```python
from build123d import *

# Parameters (mm, degrees)
F1_DEPTH = 50


with BuildPart() as f1:
    # F0 (on Front) → F1 (new body, symmetric)
    with BuildSketch(Plane.XZ):
        with BuildLine():
            ThreePointArc((34.65832, 938.949756), (117.683363, 991.882101), (150, 1084.890842))
            ThreePointArc((150, 1084.890842), (-93.008741, 1202.574206), (-34.65832, 938.949756))
            ThreePointArc((-34.65832, 938.949756), (0, 934.890842), (34.65832, 938.949756))
        make_face()
        with BuildLine():
            ThreePointArc((34.65832, 938.949756), (0, 934.890842), (-34.65832, 938.949756))
            Line((-34.65832, 938.949756), (-34.65832, 414.451611))
            Line((-34.65832, 414.451611), (-496.485632, 782.202331))
            Line((-496.485632, 782.202331), (-577.730775, 697.129786))
            Line((-577.730775, 697.129786), (-34.65832, 364.602458))
            Line((-34.65832, 364.602458), (-34.65832, -64.047714))
            Line((-34.65832, -64.047714), (-456.351271, -622.056438))
            Line((-456.351271, -622.056438), (-399.381399, -665.109158))
            Line((-399.381399, -665.109158), (-34.65832, -182.486293))
            Line((-34.65832, -182.486293), (0, -136.624381))
            Line((0, -136.624381), (34.65832, -182.486293))
            Line((34.65832, -182.486293), (399.381399, -665.109158))
            Line((399.381399, -665.109158), (456.351271, -622.056438))
            Line((456.351271, -622.056438), (34.65832, -64.047714))
            Line((34.65832, -64.047714), (34.65832, 364.602458))
            Line((34.65832, 364.602458), (577.730775, 697.129786))
            Line((577.730775, 697.129786), (496.485632, 782.202331))
            Line((496.485632, 782.202331), (34.65832, 414.451611))
            Line((34.65832, 414.451611), (34.65832, 938.949756))
        make_face()
    extrude(amount=F1_DEPTH, both=True)


solid = f1.part
```
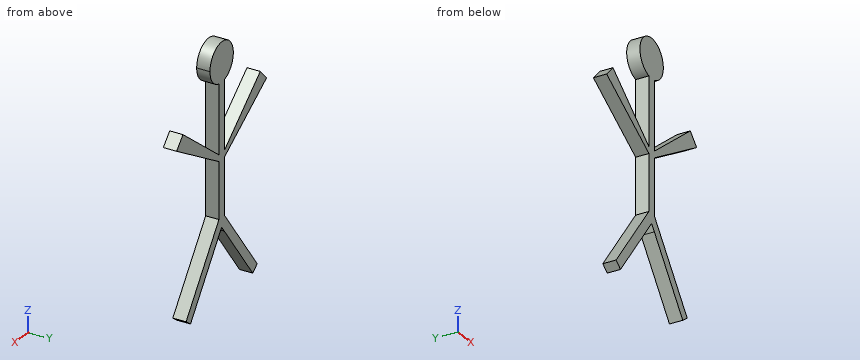
Geometry: final body of the model. Coordinates: model frame, mm. Round coordinates to 2 decimals unless told otherwise and drop trailing zeros. Order: outer loops, then holes, each group sorted by start corner. A loop starts at its lowest first (then second) coordinate and runs counter-clockwise, first axis right, second up. Notation, with made-up numbers: (32, 29.5) -> (37, 29.5) arc R28 cw to (37, 56.5) -> close; hole circle Ø3 at (-36.5, 19.5). An arc over 180 degrees is marked (long way). Write each question's results on one line, items separated by ' | '.
Q1. Ray query, line 1 along Z through (x, y) = (128, 3); line 2 along X through (y, z) = (10.5, 630); line 3 along Z through (x, y) = (-101.5, 37). Return the intervals inside material, ascending.
Response values:
line 1: -306 to -187.56, 421.76 to 488.78, 1006.69 to 1163.1 | line 2: -468.1 to -305.35, -34.66 to 34.66, 305.35 to 468.1 | line 3: -270.94 to -152.5, 405.53 to 467.68, 974.45 to 1195.33
Q2. Section query B-B (x = -420.5). Output: boundary loops of the cut face in (y, z).
Response values:
outline: (-50, -649.15) -> (50, -649.15) -> (50, -574.62) -> (-50, -574.62) -> close; (-50, 600.86) -> (50, 600.86) -> (50, 721.7) -> (-50, 721.7) -> close
Q3. Section query C-C (z = 457). Output: boundary loops of the cut face in (x, y), and give its area (3 significant figures).
Response values:
outline: (-185.56, -50) -> (-88.09, -50) -> (-88.09, 50) -> (-185.56, 50) -> close; (-34.66, -50) -> (34.66, -50) -> (34.66, 50) -> (-34.66, 50) -> close; (88.09, -50) -> (185.56, -50) -> (185.56, 50) -> (88.09, 50) -> close | area: 26,400 mm²
Q4. Section query D-D (y = 27.5). Output: boundary loops of the cut face in (x, z), and give its area (3 significant figures).
Response values:
outline: (-577.73, 697.13) -> (-34.66, 364.6) -> (-34.66, -64.05) -> (-456.35, -622.06) -> (-399.38, -665.11) -> (0, -136.62) -> (399.38, -665.11) -> (456.35, -622.06) -> (34.66, -64.05) -> (34.66, 364.6) -> (577.73, 697.13) -> (496.49, 782.2) -> (34.66, 414.45) -> (34.66, 938.95) arc R150 ccw (long way) to (-34.66, 938.95) -> (-34.66, 414.45) -> (-496.49, 782.2) -> close | area: 336,000 mm²
Q5. Section query A-A (z = -359). Output: boundary loops of the cut face in (x, y).
Response values:
outline: (-257.56, -50) -> (-168.05, -50) -> (-168.05, 50) -> (-257.56, 50) -> close; (168.05, -50) -> (257.56, -50) -> (257.56, 50) -> (168.05, 50) -> close
Q6. Pin query (flat end, axial travel): pin 1 Ø3 at (y, z) = (-40, 860.5) entering from +X; pin 2 Ø12 at (x, y) = (185, -38) entering from -Z; pin 3 Ø12 at (x, y) = (-418, 23.5) entering from +Z. Return the tip coordinate at first contact, or that it passes through.
Response values:
pin 1: x = 34.66 | pin 2: z = -389.37 | pin 3: z = 724.48
